from build123d import *

# Parameters (mm, degrees)
BOSS_EXTRUDE1_DEPTH = 4.826
FILLET1_R           = 3.175
SKETCH2_R           = 3.175
CUT_EXTRUDE1_DEPTH  = 64.68312395


with BuildPart() as part:
    # Sketch1 → Boss-Extrude1 (new body)
    with BuildSketch(Plane(origin=(0, 0, 0), x_dir=(1, 0, 0), z_dir=(0, 1, 0))):
        Polygon((-25.4, 38.1), (-25.4, 12.7), (-50.8, 12.7), (-50.8, -12.7), (-25.4, -12.7), (-25.4, -38.1), (25.4, -38.1), (25.4, 38.1), align=None)
    extrude(amount=BOSS_EXTRUDE1_DEPTH)

    # Fillet1
    fillet1_edges = [part.edges().sort_by_distance(p)[0] for p in [
        (25.4, 2.413, -38.1),
        (25.4, 2.413, 38.1),
        (-25.4, 2.413, 38.1),
        (-25.4, 2.413, 12.7),
        (-50.8, 2.413, 12.7),
        (-50.8, 2.413, -12.7),
        (-25.4, 2.413, -12.7),
        (-25.4, 2.413, -38.1),
    ]]
    fillet(fillet1_edges, radius=FILLET1_R)

    # Sketch2 → Cut-Extrude1 (cut, through all)
    with BuildSketch(Plane(origin=(0, 4.826, 0), x_dir=(1, 0, 0), z_dir=(0, 1, 0))):
        with Locations(Location((-38.1, 0, 0), (0, 0, 270))):
            Circle(SKETCH2_R)
        with Locations(Location((-12.7, 0, 0), (0, 0, 270))):
            Circle(SKETCH2_R)
    extrude(amount=-CUT_EXTRUDE1_DEPTH, mode=Mode.SUBTRACT)


solid = part.part
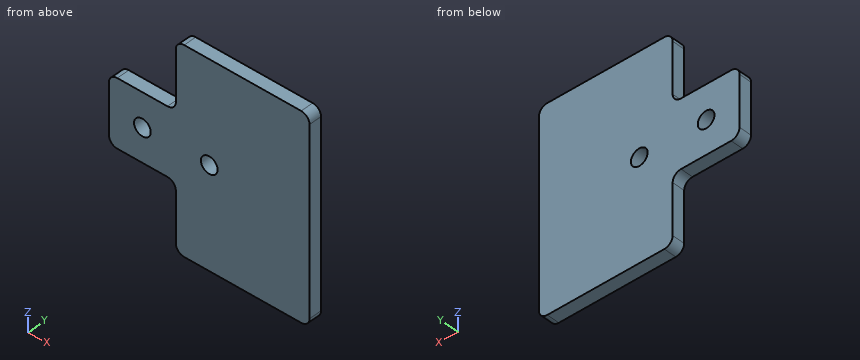
Design review of the part built by this model. Coordinates are the model's own, in mm. Give positions to 0.01 mm unless a question says otherwise; leave off trailing zeros. Loops run counter-clockwise (first coordinate to the right, second up) from the corner with the lowest first, then second, coordinate; pieces in that order, holes last. Notation, with made-up numbers: M 44.25,-35 L 53.25,-35 A6 ccw 53.25,-30 Z; hole C 59.25,30.5 d10. An arc over 180 degrees is marked long. One line per question, with ' | ' between items. Start each with the question number.
1. Add section D-D (x = -12.7). Write out the cut boundary in (y, z) (3 decimals), plus the area to 3 significant figures.
2. Add section B-B (z = 0). Write out the cut boundary in (x, y) (3 decimals), plus the area to 3 significant figures.
3. Add section A-A (x = -38.1). Write out the cut boundary in (y, z) (3 decimals).
4. Add section C-C (y = 1.9). Write out the cut boundary in (x, z) (3 decimals).
5. To check wall thickness, follow L1, parallel to X at y = 2.1, z = 0 (3 decimals); L2, parallel to X at y = 4.25, z = -2; L3, parallel to X at y = 1.15, z = -23.5. State the ranges of each line that lie inside material, in increasing order.
6. Insertion check: P1, Ø1, axis at y = 0.5, z = -26.5, coming from the -X side; P2, Ø5.5, axis at x = -12.7, z = 0, coming from the -Y side. Each pin has a flat end and moves straight along its axis. Give the tip position at first contact, or say it passes through.
Worked out:
1) outline: M 0,-38.1 L 4.826,-38.1 L 4.826,-3.175 L 0,-3.175 Z; M 0,3.175 L 4.826,3.175 L 4.826,38.1 L 0,38.1 Z | area: 337 mm²
2) outline: M -50.8,0 L -41.275,0 L -41.275,4.826 L -50.8,4.826 Z; M -34.925,0 L -15.875,0 L -15.875,4.826 L -34.925,4.826 Z; M -9.525,0 L 25.4,0 L 25.4,4.826 L -9.525,4.826 Z | area: 306 mm²
3) outline: M 0,-12.7 L 4.826,-12.7 L 4.826,-3.175 L 0,-3.175 Z; M 0,3.175 L 4.826,3.175 L 4.826,12.7 L 0,12.7 Z
4) outline: M -50.8,-9.525 A3.175 ccw -47.625,-12.7 L -28.575,-12.7 A3.175 cw -25.4,-15.875 L -25.4,-34.925 A3.175 ccw -22.225,-38.1 L 22.225,-38.1 A3.175 ccw 25.4,-34.925 L 25.4,34.925 A3.175 ccw 22.225,38.1 L -22.225,38.1 A3.175 ccw -25.4,34.925 L -25.4,15.875 A3.175 cw -28.575,12.7 L -47.625,12.7 A3.175 ccw -50.8,9.525 Z; hole C -38.1,0 d6.35; hole C -12.7,0 d6.35
5) L1: x = -50.8 to -41.275, -34.925 to -15.875, -9.525 to 25.4 | L2: x = -50.8 to -40.57, -35.63 to -15.17, -10.23 to 25.4 | L3: x = -25.4 to 25.4
6) P1: stops at x = -25.4 | P2: passes through
